Study the drawing (mm; zero at the part's minimum x, y, z) and answer. A direction names the side the tool comes from. Round coordinates to 2 decimals unless told otherwise and drop trailing zeros. Loops run counter-clockwise (first coordinate to the right, second up) from the corner with the lowest first, then second, coordinate; pieces in that order, holes last. Notation, with made-up numbers: (-19.75, 28.5) -> (-5.75, 28.5) arc R15 ccw to (-5.75, 35.5) -> close; hole circle Ø8 at (67, 33). An arc over 180 degrees is marked (long way). Write each question's results on one line, items separated by ' | '. Start each with the question number.
(1) Straight lines are drawn through the part: probe 1 along X at (y, z) = (61, 22); probe 2 along X at (y, z) = (1, 22); probe 3 along Z at (x, y) = (52.5, 62.15). For each, find the intervals that lie inside material, in ascending order.
(2) The part is cut by section A-A (x = 10). Determine the outline of the cut face in (y, z).
(3) Flat-ended cylindrical pins translate along their axes: pin 1 (6 mm diameter, centred on y = 42, z = 15.5, fed in from -X); pin 2 (6 mm diameter, centred on x = 95, z = 22.5, fed in from -Y); pin 3 (2.5 mm diameter, centred on y = 1, z = 26.5, fed in from +X). Find the tip coordinate at first contact, or state that the pin passes through.
(4) The part is cut by section D-D (z = 22.5). Count the separate pieces of the cut face and the enclosed holes in it, plus the area to 3 significant figures.
(5) The part is cut by section C-C (x = 102.5). Determine the outline of the cut face in (y, z), plus the area to 3 significant figures.
(6) For the marked faces 5, 6 and 7, determine the directions among +Z, -Z, +X, -X, +Y, -Y from which every point of the face is accessible in a straight line to the end or side of a thin tool.
(7) The part is cut by section B-B (y = 23.5). Determine the outline of the cut face in (x, z), plus the area to 3 significant figures.
(8) Determine the mould class of the marked faces 1, 2, 3 and 4 for opening direction Y: released by +Y, released by -Y, zero draft, split by the parting line, or undercut.
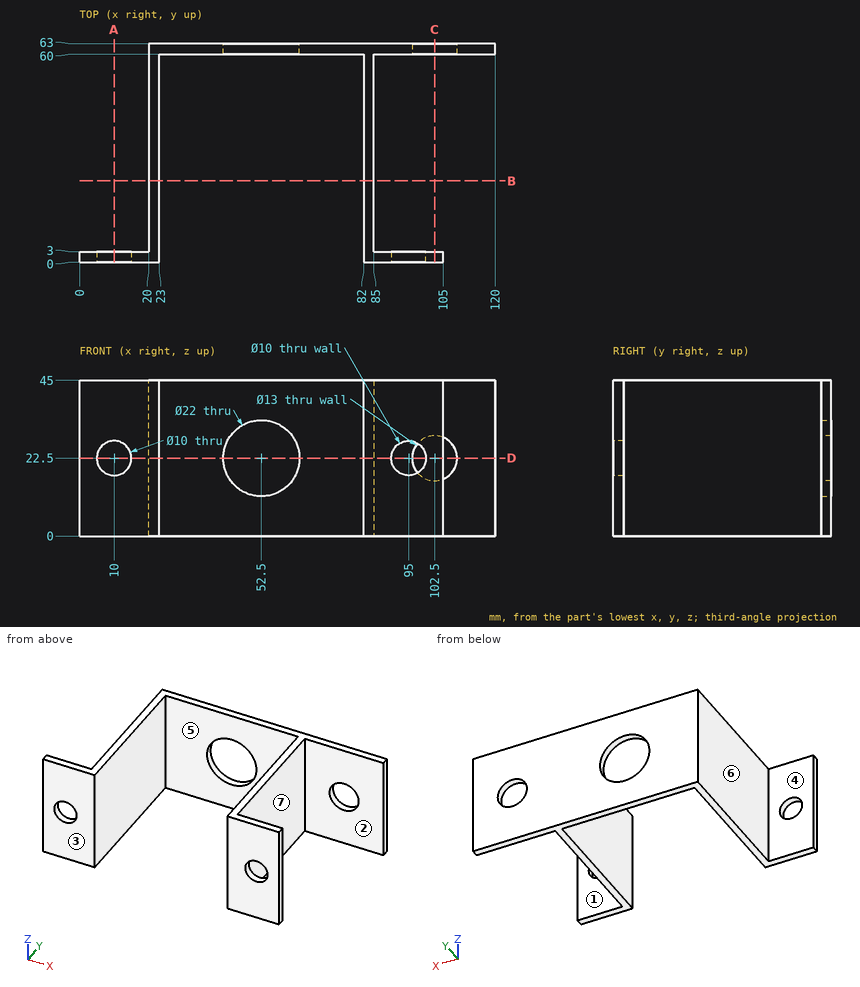
Checked values:
1) probe 1: x = 20 to 41.51, 63.49 to 96.02, 108.98 to 120 | probe 2: x = 0 to 5.03, 14.97 to 23, 82 to 90.03, 99.97 to 105 | probe 3: z = 0 to 11.5, 33.5 to 45
2) outline: (0, 0) -> (3, 0) -> (3, 17.5) -> (0, 17.5) -> close; (0, 27.5) -> (3, 27.5) -> (3, 45) -> (0, 45) -> close
3) pin 1: stops at x = 20 | pin 2: stops at y = 60 | pin 3: stops at x = 105
4) separate pieces: 5 | enclosed holes: 0 | area: 615 mm2
5) outline: (0, 0) -> (3, 0) -> (3, 45) -> (0, 45) -> close; (60, 0) -> (63, 0) -> (63, 16) -> (60, 16) -> close; (60, 29) -> (63, 29) -> (63, 45) -> (60, 45) -> close | area: 231 mm2
6) face 5: +Z, -Z, -Y | face 6: +Z, -Z, -X, +Y | face 7: +Z, -Z, +X
7) outline: (20, 0) -> (23, 0) -> (23, 45) -> (20, 45) -> close; (82, 0) -> (85, 0) -> (85, 45) -> (82, 45) -> close | area: 270 mm2
8) face 1: undercut | face 2: undercut | face 3: released by -Y | face 4: released by +Y
